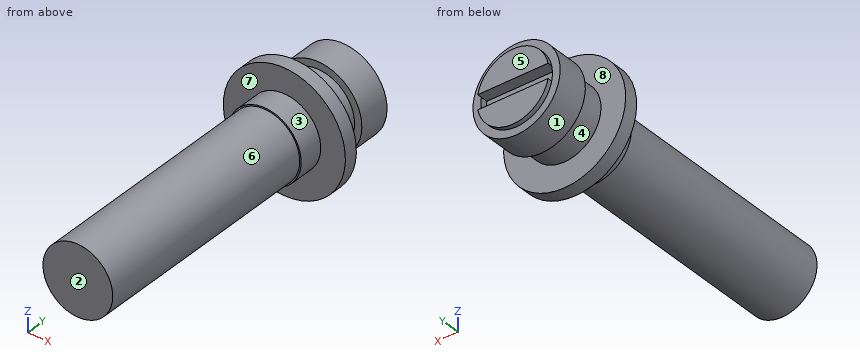
from build123d import *

# Parameters (mm, degrees)
ENL_V_START             = -2
ENL_V_MAT_EXTRU_1_DEPTH = 2


with BuildPart() as part:
    # Esquisse2 → Révolution1 (revolve)
    with BuildSketch(Plane.XY, mode=Mode.PRIVATE) as r_volution1_sk:
        Polygon((0, 64.893975029), (6.175, 64.893975029), (6.175, 64.093975029), (7.5, 64.093975029), (7.5, 58.593975029), (6.25, 58.593975029), (6.25, 53.593975029), (10.5, 53.593975029), (10.5, 51.193975029), (6.25, 51.193975029), (6.25, 46.933975029), (6, 46.933975029), (6, 6.093975029), (0, 6.093975029), align=None)
    revolve(r_volution1_sk.sketch.rotate(Axis((0, 0, 0), (0, 1, 0)), 90), axis=Axis((0, 0, 0), (0, 1, 0)))

    # Esquisse3 → Enlèv. mat.-Extru.1 (cut)
    with BuildSketch(Plane(origin=(0, 64.893975029, 0), x_dir=(1, 0, 0), z_dir=(0, 1, 0)).offset(ENL_V_START)):
        with BuildLine():
            Line((-6.047158424, 1.25), (6.047158424, 1.25))
            ThreePointArc((6.047158424, 1.25), (6.175, 0), (6.047158424, -1.25))
            Line((6.047158424, -1.25), (-6.047158424, -1.25))
            ThreePointArc((-6.047158424, -1.25), (-6.175, 0), (-6.047158424, 1.25))
        make_face()
    extrude(amount=ENL_V_MAT_EXTRU_1_DEPTH, mode=Mode.SUBTRACT)


solid = part.part
Geometry: final body of the model. Coordinates: model frame, mm. Face numbers are marked on the shaded views. A direction names the side the tool comes from. Give positions to 0.01 mm unless a question says otherwise; leave off trailing zeros. Loops run counter-clockwise (first coordinate to the right, second up) from the corner with the lowest first, then second, coordinate; pieces in that order, holes last. Notation, with made-up numbers: M -31,81 L -18,81 A21 cw -18,87 Z; hole C -16,83 d6. An arc over 180 degrees is marked long. Put each result on its own line as item: value. Start each with the question number.
1) Ray query, line 1 along Y through (x, z) = (0.5, 7); line 2 along Y through (x, z) = (3.5, 0.5); line 3 along Y through (x, z) = (-9.5, -2.5). Return the intervals inside material, ascending.
2) Contact query for flat-ended pins moving along their axis: pin 1 (2 mm diameter, centred on x = -1.5, y = 20, fed in from +Z); pin 2 (2 mm diameter, centred on x = -2, y = 64, fed in from -Z); pin 3 (6 mm diameter, centred on x = -7.5, y = 33.5, fed in from +Z). Output: stop coordinate, or through.
3) Pull-direction query (Y, two-part tool) for the marked faces 5, 6, 7 and 8; classes: pulls with the +Y half, pulls with the -Y half, needs draft (parallel to the pull), parting line crosses it, or undercut.
4) Cut plane A-A (x = 0). Output: boundary loops of the cut face in (y, z) (3 decimals), then the cut area to 3 significant figures.
5) Cut plane D-D (y = 37). Output: boundary loops of the cut face in (x, z), then the cut area to 3 significant figures.
6) Cut plane C-C (y = 49.5). Output: boundary loops of the cut face in (x, z), then the cut area to 3 significant figures.
7) Cut plane B-B (z = 0). Output: boundary loops of the cut face in (x, y) (3 decimals), then the cut area to 3 significant figures.
8) Access query for the marked faces 1, 2, 3 and 4. Directions: +Z, -Z, +X, -X, +Y, -Y. A direction counts if a zero-diameter tool reaches every point of the face in a straight line with its end or side. Return the directions, or none.
Verdict:
1. line 1: 51.19 to 53.59, 58.59 to 64.09
1. line 2: 6.09 to 62.89
1. line 3: 51.19 to 53.59
2. pin 1: z = 5.98
2. pin 2: z = -7.43
2. pin 3: z = 3.97
3. face 5: pulls with the +Y half
3. face 6: needs draft
3. face 7: pulls with the -Y half
3. face 8: undercut
4. outline: M 6.094,-6 L 46.934,-6 L 46.934,-6.25 L 51.194,-6.25 L 51.194,-10.5 L 53.594,-10.5 L 53.594,-6.25 L 58.594,-6.25 L 58.594,-7.5 L 64.094,-7.5 L 64.094,-6.175 L 64.894,-6.175 L 64.894,-1.25 L 62.894,-1.25 L 62.894,1.25 L 64.894,1.25 L 64.894,6.175 L 64.094,6.175 L 64.094,7.5 L 58.594,7.5 L 58.594,6.25 L 53.594,6.25 L 53.594,10.5 L 51.194,10.5 L 51.194,6.25 L 46.934,6.25 L 46.934,6 L 6.094,6 Z
4. area: 744 mm2
5. outline: C 0,0 d12
5. area: 113 mm2
6. outline: C 0,0 d12.5
6. area: 123 mm2
7. outline: M -10.5,51.194 L -6.25,51.194 L -6.25,46.934 L -6,46.934 L -6,6.094 L 6,6.094 L 6,46.934 L 6.25,46.934 L 6.25,51.194 L 10.5,51.194 L 10.5,53.594 L 6.25,53.594 L 6.25,58.594 L 7.5,58.594 L 7.5,64.094 L 6.175,64.094 L 6.175,62.894 L -6.175,62.894 L -6.175,64.094 L -7.5,64.094 L -7.5,58.594 L -6.25,58.594 L -6.25,53.594 L -10.5,53.594 Z
7. area: 724 mm2
8. face 1: +Y
8. face 2: +Z, -Z, +X, -X, -Y
8. face 3: -Y
8. face 4: none
